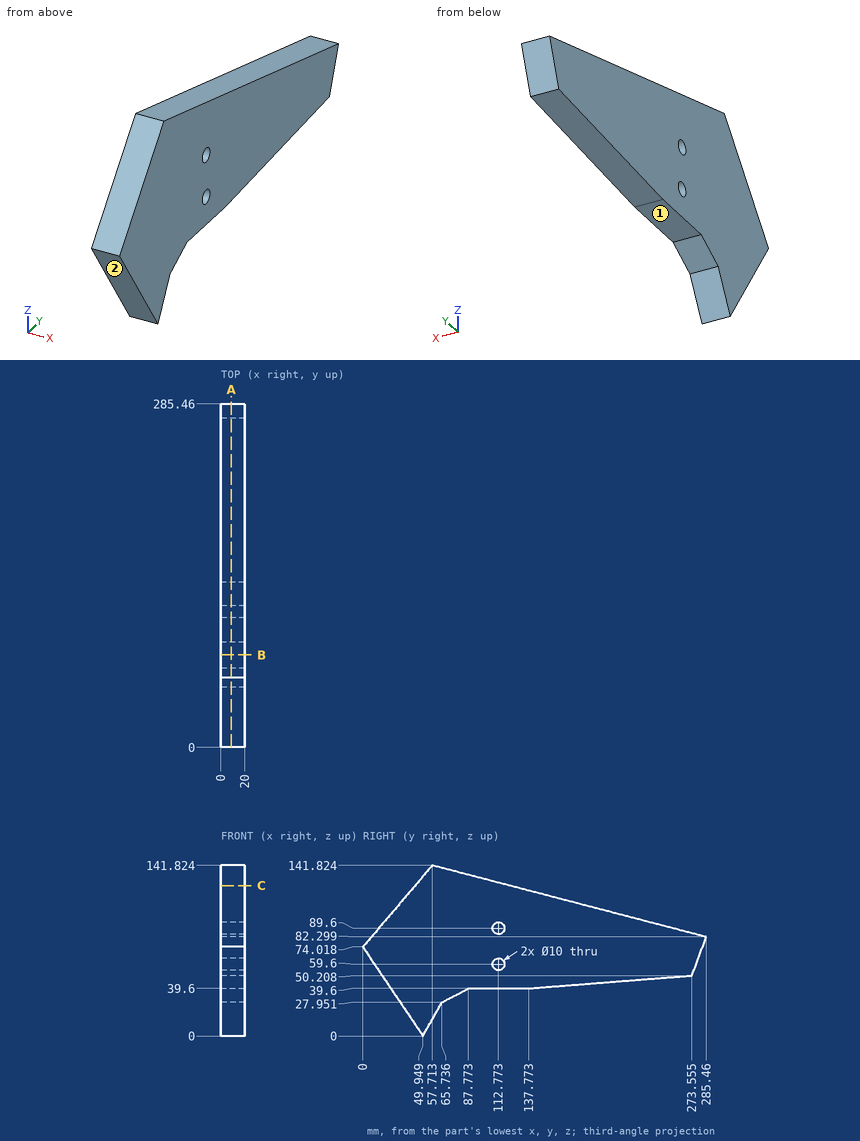
Design review of the part shown in the three views and the two pictorial views. Dimensions are in mm from the part's minimum x, y and z. A direction names the side the tool comes from. Round coordinates to 2 decimals unless told otherwise and drop trailing zeros. Loops run counter-clockwise (first coordinate to the right, second up) from the corner with the lowest first, then second, coordinate; pieces in that order, holes last. Notation, with made-up numbers: (35, 21.25) - (47, 21.25) arc R20 cw to (47, 45.25) - close; hole circle Ø1 at (46, 4). An arc over 180 degrees is marked (long way). Use one line per item in the form item = value.
1) We need section A-A on x = 8.75. State how many separate pieces and enclosed holes the cut face has, then the cut area to 3 significant figures.
Solutions:
separate_pieces = 1
enclosed_holes = 2
area = 19,900 mm2
2) Clearance check with flat-ended pins moving along their axes: P1, Ø8, axis at y = 112.77, z = 59.6, coming from the -X side; P2, Ø10, axis at x = 9, y = 100, coming from the +Z side; P3, Ø5, axis at x = 12.5, z = 39, coming from the -Y side (1 decimal); P4, Ø6, axis at x = 7, y = 135, coming from the +Z side. State where each tip first meets the part, or that it passes through.
Solutions:
P1 = through
P2 = 132.08
P3 = 21.9
P4 = 122.41
3) We need section C-C on z = 125. Write out the cut boundary in (x, y).
Solutions:
outline = (0, 43.39) - (20, 43.39) - (20, 122.08) - (0, 122.08) - close
4) Wall thickness on probe 1 along Z at (x, y) = (16.25, 232); probe 2 along Z at (x, y) = (12, 128.5); probe 3 along Y at (x, z) = (18.75, 70) (1 decimal): over which ranges is each line inside the solid? List them lowest first.
Solutions:
probe_1 = 46.96 to 96.27
probe_2 = 39.6 to 123.32
probe_3 = 2.7 to 280.9
5) We need section B-B on y = 77. Write out the cut boundary in (x, z) (1 decimal), then the cut area to 3 significant figures.
Solutions:
outline = (0, 33.9) - (20, 33.9) - (20, 136.8) - (0, 136.8) - close
area = 2,060 mm2
6) Tool access review of the marked faces 1 and 2: name each direction out of +Z, -Z, +X, -X, +Y, -Y from which nothing blocks a thin tool from reaching the whole face with its end or side.
Solutions:
face_1 = -Z, +X, -X, +Y
face_2 = -Z, +X, -X, -Y
